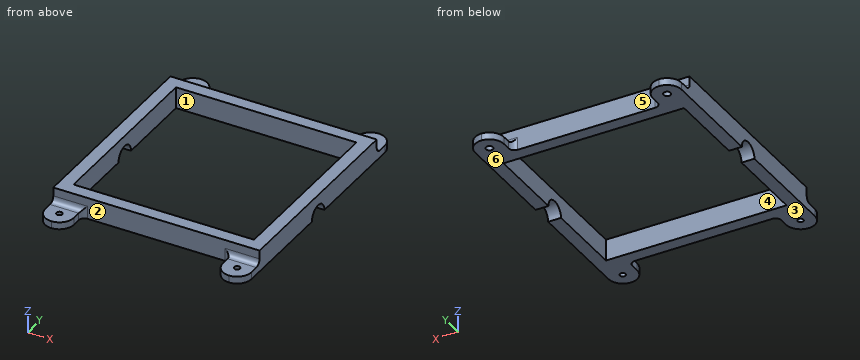
from build123d import *

# Parameters (mm, degrees)
SKETCH1_W            = 91.44
SKETCH1_H            = 91.44
BOSS_EXTRUDE1_DEPTH  = 9.525
SKETCH2_W            = 80.01
SKETCH2_H            = 80.01
CUT_EXTRUDE1_DEPTH   = 9.525
SKETCH3_R            = 4.8895
CUT_EXTRUDE2_DEPTH   = 103.675788894
SKETCH4_W            = 12.7
SKETCH4_H            = 12.7
BOSS_EXTRUDE2_DEPTH  = 3.175
SKETCH5_R            = 1.5875
CUT_EXTRUDE3_DEPTH   = 75.454934692
FILLET1_R            = 6.35
FILLET2_R            = 2.54
FILLET1_OF_MIRROR1_R = 6.35
FILLET2_OF_MIRROR1_R = 2.54
SKETCH6_W            = 12.7
SKETCH6_H            = 12.7
SKETCH6_R            = 1.27
BOSS_EXTRUDE3_DEPTH  = 3.175
FILLET3_R            = 2.54
FILLET4_R            = 6.35
FILLET3_OF_MIRROR7_R = 2.54
FILLET4_OF_MIRROR7_R = 6.35


with BuildPart() as part:
    # Sketch1 → Boss-Extrude1 (new body)
    with BuildSketch(Plane.XY):
        Rectangle(SKETCH1_W, SKETCH1_H)
    extrude(amount=BOSS_EXTRUDE1_DEPTH)

    # Sketch2 → Cut-Extrude1 (cut)
    with BuildSketch(Plane.XY.offset(9.525)):
        Rectangle(SKETCH2_W, SKETCH2_H)
    extrude(amount=-CUT_EXTRUDE1_DEPTH, mode=Mode.SUBTRACT)

    # Sketch3 → Cut-Extrude2 (cut, through all)
    with BuildSketch(Plane(origin=(45.72, 0, 0), x_dir=(0, 0, -1), z_dir=(1, 0, 0))):
        Circle(SKETCH3_R)
        with Locations((0, 57.404)):
            Circle(SKETCH3_R)
        with Locations((0, -57.404)):
            Circle(SKETCH3_R)
    extrude(amount=-CUT_EXTRUDE2_DEPTH, mode=Mode.SUBTRACT)

    # Sketch4 → Boss-Extrude2 (add)
    with BuildSketch(Plane(origin=(0, 0, 0), x_dir=(-1, 0, 0), z_dir=(0, 0, -1))):
        with Locations((-39.37, 52.07)):
            Rectangle(SKETCH4_W, SKETCH4_H)
    boss_extrude2 = extrude(amount=-BOSS_EXTRUDE2_DEPTH)

    # Sketch5 → Cut-Extrude3 (cut, through all)
    with BuildSketch(Plane.XY.offset(3.175)):
        with Locations((39.37, 52.07)):
            Circle(SKETCH5_R)
    cut_extrude3 = extrude(amount=-CUT_EXTRUDE3_DEPTH, mode=Mode.SUBTRACT)

    # Fillet1
    fillet1_edges = [part.edges().sort_by_distance(p)[0] for p in [
        (33.02, 58.42, 1.5875),
        (45.72, 58.42, 1.5875),
    ]]
    fillet(fillet1_edges, radius=FILLET1_R - 0.0001)  # a hair under: the kernel refuses the full size

    # Fillet2
    fillet2_edges = [part.edges().sort_by_distance(p)[0] for p in [
        (39.37, 45.72, 3.175),
        (33.02, 45.72, 1.5875),
    ]]
    fillet(fillet2_edges, radius=FILLET2_R)

    # Mirror1: Boss-Extrude2, Cut-Extrude3 across plane
    add(boss_extrude2.mirror(Plane(origin=(0, 0, 0), x_dir=(0, 0, 1), z_dir=(1, 0, 0))))
    add(cut_extrude3.mirror(Plane(origin=(0, 0, 0), x_dir=(0, 0, 1), z_dir=(1, 0, 0))), mode=Mode.SUBTRACT)

    # Fillet1 of Mirror1
    fillet1_of_mirror1_edges = [part.edges().sort_by_distance(p)[0] for p in [
        (-33.02, 58.42, 1.5875),
        (-45.72, 58.42, 1.5875),
    ]]
    fillet(fillet1_of_mirror1_edges, radius=FILLET1_OF_MIRROR1_R - 0.0001)  # a hair under: the kernel refuses the full size

    # Fillet2 of Mirror1
    fillet2_of_mirror1_edges = [part.edges().sort_by_distance(p)[0] for p in [
        (-39.37, 45.72, 3.175),
        (-33.02, 45.72, 1.5875),
    ]]
    fillet(fillet2_of_mirror1_edges, radius=FILLET2_OF_MIRROR1_R)

    # Sketch6 → Boss-Extrude3 (add)
    with BuildSketch(Plane(origin=(0, 0, 0), x_dir=(-1, 0, 0), z_dir=(0, 0, -1))):
        with Locations((-39.37, -52.07)):
            Rectangle(SKETCH6_W, SKETCH6_H)
        with Locations((-39.37, -52.07)):
            Circle(SKETCH6_R, mode=Mode.SUBTRACT)
    boss_extrude3 = extrude(amount=-BOSS_EXTRUDE3_DEPTH)

    # Fillet3
    fillet3_edges = [part.edges().sort_by_distance(p)[0] for p in [
        (39.37, -45.72, 3.175),
        (33.02, -45.72, 1.5875),
    ]]
    fillet(fillet3_edges, radius=FILLET3_R)

    # Fillet4
    fillet4_edges = [part.edges().sort_by_distance(p)[0] for p in [
        (45.72, -58.42, 1.5875),
        (33.02, -58.42, 1.5875),
    ]]
    fillet(fillet4_edges, radius=FILLET4_R - 0.0001)  # a hair under: the kernel refuses the full size

    # Mirror7: Boss-Extrude3 across plane
    add(boss_extrude3.mirror(Plane(origin=(0, 0, 0), x_dir=(0, 0, 1), z_dir=(1, 0, 0))))

    # Fillet3 of Mirror7
    fillet3_of_mirror7_edges = [part.edges().sort_by_distance(p)[0] for p in [
        (-39.37, -45.72, 3.175),
        (-33.02, -45.72, 1.5875),
    ]]
    fillet(fillet3_of_mirror7_edges, radius=FILLET3_OF_MIRROR7_R)

    # Fillet4 of Mirror7
    fillet4_of_mirror7_edges = [part.edges().sort_by_distance(p)[0] for p in [
        (-45.72, -58.42, 1.5875),
        (-33.02, -58.42, 1.5875),
    ]]
    fillet(fillet4_of_mirror7_edges, radius=FILLET4_OF_MIRROR7_R - 0.0001)  # a hair under: the kernel refuses the full size


solid = part.part
The model under review builds one solid part; all positions refer to its coordinate system, in mm. Face numbers are marked on the shaded views. A direction names the side the tool comes from. Give positions to 0.01 mm unless a question says otherwise; leave off trailing zeros. Write each loop counter-clockwise with the first axis right and the second up, starting at its lowest first coordinate (ties: lowest second). Pieces come first, ordered by that corner, then holes.
1. Draft analysis for pull direction Y (two halves, no side actions). For the marked faces 1, 2 and 3, state which applies: +Y half, -Y half, draft (parallel to the pull), parting line (faces both ways), or undercut.
2. Add section B-B, the plane x = 3. Write out the cut boundary in (y, z) (3 decimals).
3. Tool access review of the marked faces 4, 5 and 6: name each direction out of +Z, -Z, +X, -X, +Y, -Y from which nothing blocks a thin tool from reaching the whole face with its end or side.
4. Add section C-C, the plane z = 7. Write out the cut boundary in (x, y) (3 decimals), plus the area to 3 significant figures.
5. Add section A-A, the plane y = 0. Write out the cut boundary in (x, z) (1 decimal).
6. Wall thickness on L1, parallel to Y at x = 39.37, z = 2.25 (1 decimal); L2, parallel to X at y = 7.5, z = 7.25 (3 decimals): over which ranges is each line inside the solid? List them lowest first.
7. For P1, Ø1.5, axis at x = 14, z = 4.5, coming from the -Y side; P2, Ø5, axis at x = -32, z = 1, coming from the +Y side; P3, Ø5, axis at x = -38, y = -54, coming from the +Z side (3 decimals); P4, Ø2.5, axis at x = -39.37, y = 52.07, coming from the +Z side, all flat-tipped, find the tip position at first contact; note any pin that passes through.
Worked answers:
1. face 1: undercut
1. face 2: -Y half
1. face 3: draft
2. outline: (-45.72, 0) - (-40.005, 0) - (-40.005, 9.525) - (-45.72, 9.525) - close; (40.005, 0) - (45.72, 0) - (45.72, 9.525) - (40.005, 9.525) - close
3. face 4: +Z, -Z
3. face 5: +Z, +Y
3. face 6: -Z, +X, -X, +Y, -Y
4. outline: (-45.72, -45.72) - (45.72, -45.72) - (45.72, 45.72) - (-45.72, 45.72) - close; hole (-40.005, -40.005) - (40.005, -40.005) - (40.005, 40.005) - (-40.005, 40.005) - close
4. area: 1,960 mm2
5. outline: (-45.7, 4.9) - (-40, 4.9) - (-40, 9.5) - (-45.7, 9.5) - close; (40, 4.9) - (45.7, 4.9) - (45.7, 9.5) - (40, 9.5) - close
6. L1: y = -58.4 to -53.3, -50.8 to -40, 40 to 50.5, 53.7 to 58.4
6. L2: x = -45.72 to -40.005, 40.005 to 45.72
7. P1: stops at y = -45.72
7. P2: stops at y = 56.15
7. P3: stops at z = 3.175
7. P4: passes through
